```python
from build123d import *

# Parameters (mm, degrees)
F0_R     = 3.2
F1_DEPTH = 2.4


with BuildPart() as f1:
    # F0 (on Top) → F1 (new body)
    with BuildSketch(Plane.XY):
        Polygon((43.1, 5), (43.1, 20), (22.5, 20), (22.5, 22.4), (12.5, 22.4), (12.5, 20), (-12.5, 20), (-12.5, 22.4), (-22.5, 22.4), (-22.5, 20), (-43.1, 20), (-43.1, 5), (-45.5, 5), (-45.5, -5), (-43.1, -5), (-43.1, -20), (-22.5, -20), (-22.5, -22.4), (-12.5, -22.4), (-12.5, -20), (12.5, -20), (12.5, -22.4), (22.5, -22.4), (22.5, -20), (43.1, -20), (43.1, -5), (45.5, -5), (45.5, 5), align=None)
        Polygon((-36.31, -12.67), (-36.31, -10.48), (-27.56, -10.48), (-27.56, -12.67), (-28.97, -14.08), (-34.9, -14.08), align=None, mode=Mode.SUBTRACT)
        Polygon((-18.5, -11.51), (-18.5, -6.68), (-2.5, -6.68), (-2.5, -11.51), (-5.07, -14.08), (-15.93, -14.08), align=None, mode=Mode.SUBTRACT)
        with Locations((10.9, -10.9)):
            Circle(F0_R, mode=Mode.SUBTRACT)
    extrude(amount=F1_DEPTH)


solid = f1.part
```
Design review of the part built by this model. Coordinates are the model's own, in mm. A direction names the side the tool comes from. Round coordinates to 2 decimals unless told otherwise and drop trailing zeros. Order: outer loops, then holes, each group sorted by start corner. A loop starts at its lowest first (then second) coordinate and runs counter-clockwise, first axis right, second up. Notation, with made-up numbers: (-17.5, 46) - (-7.5, 46) arc R21 ccw to (-7.5, 75) - close; hole circle Ø1 at (5, 83). An arc over 180 degrees is marked (long way). Return JSON: item names as keys, results as strings.
Q1. Consider section B-B on z = 0.9. Give the number of separate pieces and of enclosed holes in the cut face, plus the area to 3 significant figures.
Computed values:
{"separate pieces": "1", "enclosed holes": "3", "area": "3,420 mm2"}
Q2. Machinability: for faces 1 (the flat face through (-43.1, 13, 1)), 2 (the flat face through (44, -5, 1)), 3 (the flat face through (-33, -20, 1)), 4 (the flat face through (-32, -14.08, 1)), which of the approach directions +Z, -Z, +X, -X, +Y, -Y give a long, thin tool a straight path to every point of the face, cutting with its end or side? Answer none if there is none.
Computed values:
{"face 1": "+Z, -Z, -X, +Y", "face 2": "+Z, -Z, +X, -Y", "face 3": "+Z, -Z, -X, -Y", "face 4": "+Z, -Z"}
Q3. Consider section C-C on x = 10.9. Write out the cut boundary in (y, z).
Computed values:
{"outline": "(-20, 0) - (-14.1, 0) - (-14.1, 2.4) - (-20, 2.4) - close; (-7.7, 0) - (20, 0) - (20, 2.4) - (-7.7, 2.4) - close"}
Q4. Consider section A-A on x = -10.5. Write out the cut boundary in (y, z), plus the area to 3 significant figures.
Computed values:
{"outline": "(-20, 0) - (-14.08, 0) - (-14.08, 2.4) - (-20, 2.4) - close; (-6.68, 0) - (20, 0) - (20, 2.4) - (-6.68, 2.4) - close", "area": "78.2 mm2"}
Q5. The part is to be moulded in two halves that separate along X. For faces 5 (the flat face through (44, 5, 1)), 6 (the flat face through (-12.5, -21, 1)), 7 (the flat face through (45.5, 0, 1)), 8 (the flat face through (-45.5, 0, 1)), say which applies: pulls with the +X half, pulls with the -X half, needs draft (parallel to the pull), parting line crosses it, or undercut.
Computed values:
{"face 5": "needs draft", "face 6": "undercut", "face 7": "pulls with the +X half", "face 8": "pulls with the -X half"}
Q6. Consider section D-D on y = 16. Write out the cut boundary in (x, z).
Computed values:
{"outline": "(-43.1, 0) - (43.1, 0) - (43.1, 2.4) - (-43.1, 2.4) - close"}
Q7. For pin 1 Ø1.2 at (y, z) = (-21.5, 1) entering from -X; pin 2 Ø1.2 at (x, z) = (-31.5, 1) entering from -Y; pin 3 Ø0.7 at (x, z) = (32.5, 2) entering from +Y, all flat-tipped, find the tip position at first contact; note any pin that passes through.
Computed values:
{"pin 1": "stops at x = -22.5", "pin 2": "stops at y = -20", "pin 3": "stops at y = 20"}
Q8. Wall thickness on L1, parallel to X at y = -11, z = 0.8; L2, parallel to Y at x = 10.9, z = 0.75; L3, parallel to X at y = -17, z = 1.6: over which ranges is each line inside the solid? List them lowest first. Write a range as [from, to].
Computed values:
{"L1": "x = [-43.1, -36.31], [-27.56, -18.5], [-2.5, 7.7], [14.1, 43.1]", "L2": "y = [-20, -14.1], [-7.7, 20]", "L3": "x = [-43.1, 43.1]"}
